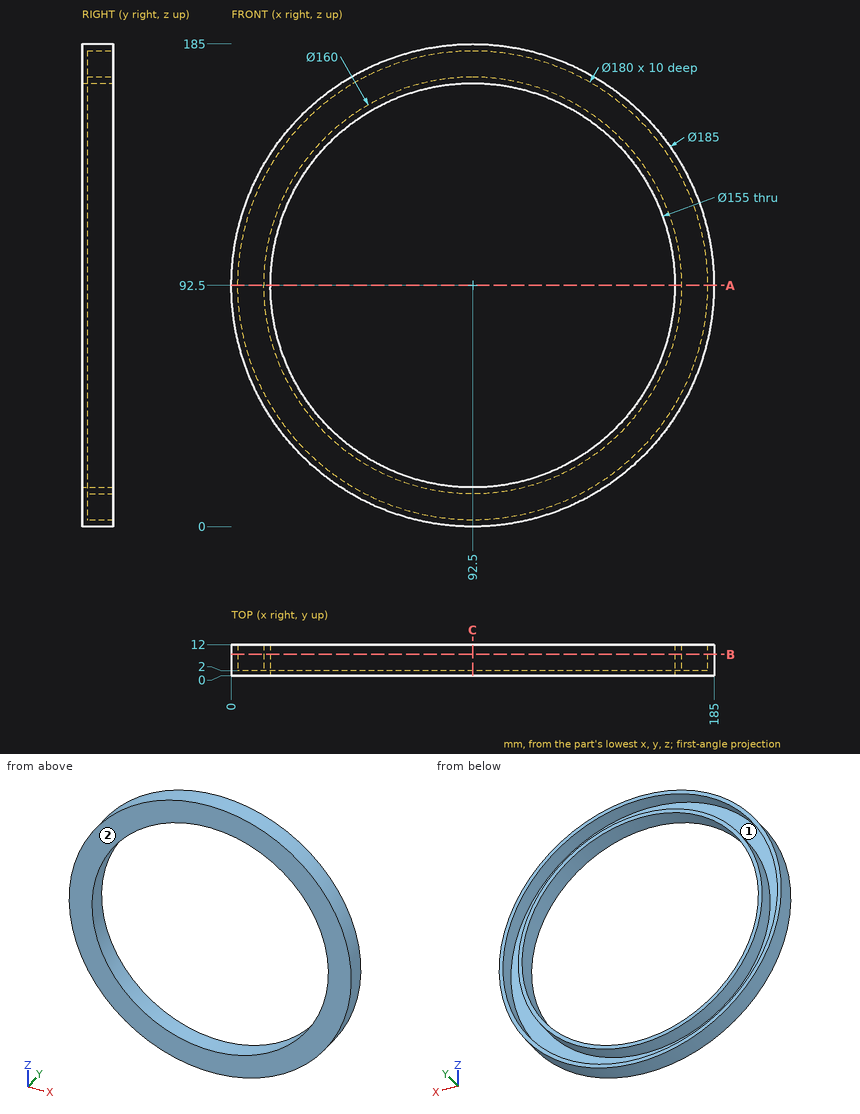
Here's the drawing with two shaded views (mm, measured from the low corner). I have some questions. Give positions to 0.01 mm unless a question says otherwise; leave off trailing zeros. Write each loop counter-clockwise with the first axis right and the second up, starting at its lowest first coordinate (ties: lowest second). Pieces come first, ordered by that corner, then holes. Notation, with made-up numbers: (9.25, 78.5) - (66.25, 78.5) arc R23 cw to (66.25, 103.5) - close; hole circle Ø3 at (78.25, -35). An arc over 180 degrees is marked (long way). Write item = value, one per line. Start each with the question number.
1. Imagine slicing it at A-A (z = 92.5). Please give me the cut outline in (x, y), and give its area (3 significant figures).
2. Imagine slicing it at B-B (y = 8.25). Please give me the cut outline in (x, z), and give its area (3 significant figures).
3. Thinking about a two-plate mould opening in Z: for the marked faces 1 and 2, which applies, released by +Z, released by -Z, zero draft, split by the parting line, or undercut?
4. For pin 1 (3 mm diameter, centred on x = 112, y = 8.5, fed in from -Z); pin 2 (6 mm diameter, centred on x = 106, y = 10.5, fed in from +Z); pin 3 (1 mm diameter, centred on x = 37, y = 10.5, fed in from +Z), each with a flat end and sliding along its axis, tell me the tip position at first contact or that it passes through.
5. Please list where these lines run through material, in increasing order: line 1 (X direction, y = 8.25, z = 92.5); line 2 (X direction, y = 7.5, z = 60.5); line 3 (Z direction, x = 154.5, y = 10).
6. Imagine slicing it at C-C (x = 92.5). Please give me the cut outline in (y, z), and give its area (3 significant figures).
Worked answers:
q1.outline = (0, 0) - (15, 0) - (15, 12) - (12.5, 12) - (12.5, 2) - (2.5, 2) - (2.5, 12) - (0, 12) - close; (170, 0) - (185, 0) - (185, 12) - (182.5, 12) - (182.5, 2) - (172.5, 2) - (172.5, 12) - (170, 12) - close
q1.area = 160 mm2
q2.outline = circle Ø185 at (92.5, 92.5); circle Ø160 at (92.5, 92.5); hole circle Ø180 at (92.5, 92.5); hole circle Ø155 at (92.5, 92.5)
q2.area = 2,670 mm2
q3.face_1 = undercut
q3.face_2 = zero draft
q4.pin_1 = 1.77
q4.pin_2 = 184.4
q4.pin_3 = 166.87
q5.line_1 = 0 to 2.5, 12.5 to 15, 170 to 172.5, 182.5 to 185
q5.line_2 = 5.71 to 8.38, 19.18 to 21.91, 163.09 to 165.82, 176.62 to 179.29
q5.line_3 = 23.85 to 27.26, 41.94 to 46, 139 to 143.06, 157.74 to 161.15
q6.outline = (0, 0) - (12, 0) - (12, 2.5) - (2, 2.5) - (2, 12.5) - (12, 12.5) - (12, 15) - (0, 15) - close; (0, 170) - (12, 170) - (12, 172.5) - (2, 172.5) - (2, 182.5) - (12, 182.5) - (12, 185) - (0, 185) - close
q6.area = 160 mm2
